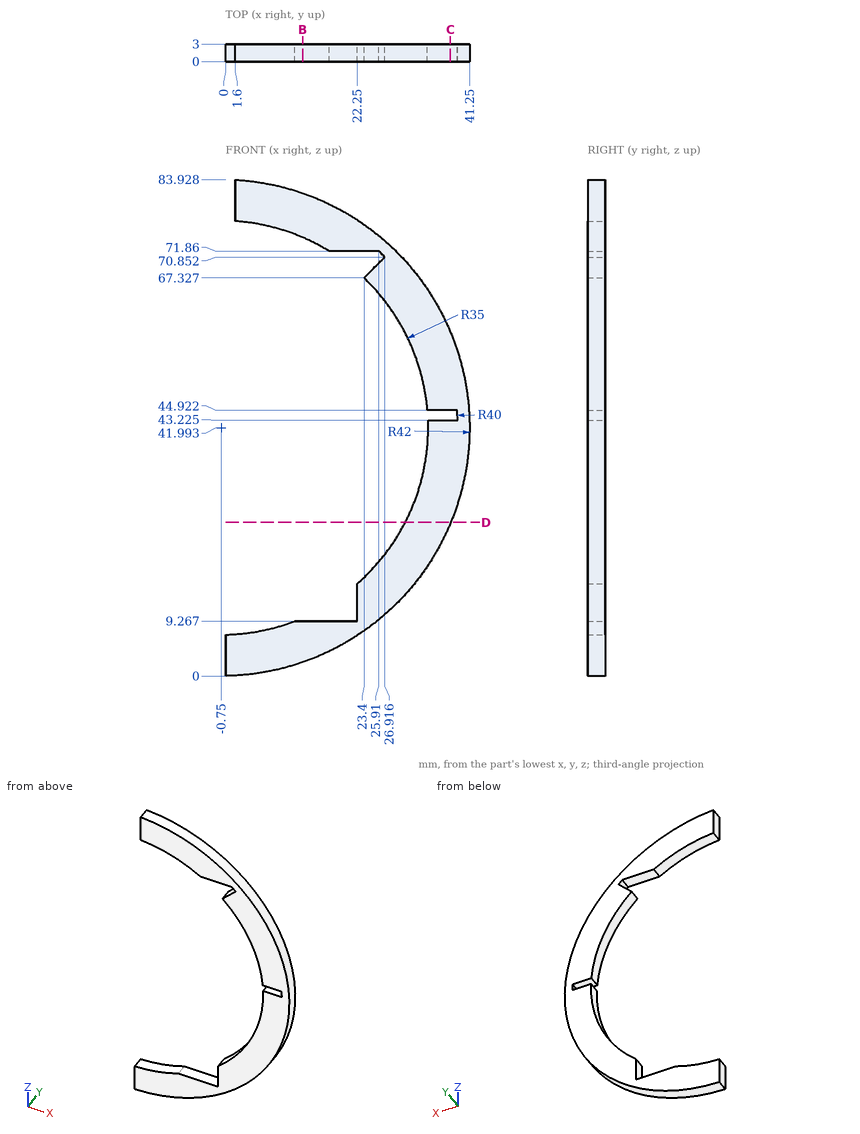
Source: three-view drawing plus pictorial views. Frame: mm from the lowest corner of the part. Give positions to 0.01 mm unless a question says otherwise; leave off trailing zeros. Write each loop counter-clockwise with the first axis right and the second up, starting at its lowest first coordinate (ties: lowest second). Pieces come first, ordered by that corner, then holes. Notation, with made-up numbers: (75, 16) - (106, 16) arc R22 ccw to (106, 36) - close; hole circle Ø5 at (-21, 40.25). An arc over 180 degrees is marked (long way). Write item = value, one per line. Start each with the question number.
Q1. Material intervals for probe 1 along Z at (x, y) = (6.5, 1.1) (1 decimal); probe 2 along Z at (x, y) = (31, 2.2) (1 decimal); probe 3 along Z at (x, y) = (24.5, 2.85) (1 decimal), sorted ascending.
Q2. Cut plane C-C, the plane x = 38. Return loops of the section in (y, z) (1 decimal).
Q3. Cut plane B-B, the plane x = 13. Return loops of the section in (y, z).
Q4. Pin query (flat end, axial travel): pin 1 Ø10 at (x, z) = (30.5, 33) entering from +Y; pin 2 Ø0.9 at (x, y) = (36.5, 1.5) entering from -Z; pin 3 Ø1.5 at (y, z) = (1, 13) entering from -X. Return the tip coordinate at first contact, or that it passes through.
Q5. Cut plane D-D, the plane z = 26. Return loops of the section in (x, y) (1 decimal).
Computed values:
q1.probe_1 = 0.6 to 7.8, 76.2 to 83.4
q1.probe_2 = 14.5 to 27.3, 56.7 to 69.5
q1.probe_3 = 8.4 to 17.8, 66.2 to 68.4, 71.9 to 75.6
q2.outline = (0, 25.8) - (3, 25.8) - (3, 43.2) - (0, 43.2) - close; (0, 44.9) - (3, 44.9) - (3, 58.2) - (0, 58.2) - close
q3.outline = (0, 2.31) - (3, 2.31) - (3, 9.27) - (0, 9.27) - close; (0, 74.18) - (3, 74.18) - (3, 81.68) - (0, 81.68) - close
q4.pin_1 = 3
q4.pin_2 = 21.75
q4.pin_3 = 22.25
q5.outline = (30.4, 0) - (38.1, 0) - (38.1, 3) - (30.4, 3) - close
